```python
from build123d import *

# Parameters (mm, degrees)
F1_DEPTH = 25


with BuildPart() as f1:
    # F0 (on Front) → F1 (new body)
    with BuildSketch(Plane.XZ):
        with BuildLine():
            ThreePointArc((0, 2), (0.5857864376, 0.5857864376), (2, 0))
            Line((2, 0), (14, 0))
            Line((14, 0), (14, 1))
            Line((14, 1), (15, 1))
            Line((15, 1), (15, 6))
            Line((15, 6), (9.95, 6))
            Line((9.95, 6), (9.95, 8.5))
            Line((9.95, 8.5), (13.95, 12.5))
            Line((13.95, 12.5), (19.5, 12.5))
            Line((19.5, 12.5), (20, 13))
            Line((20, 13), (20.5, 12.5))
            Line((20.5, 12.5), (26.05, 12.5))
            Line((26.05, 12.5), (30.05, 8.5))
            Line((30.05, 8.5), (30.05, 6))
            Line((30.05, 6), (25, 6))
            Line((25, 6), (25, 1))
            Line((25, 1), (26, 1))
            Line((26, 1), (26, 0))
            Line((26, 0), (38, 0))
            ThreePointArc((38, 0), (39.4142135624, 0.5857864376), (40, 2))
            Line((40, 2), (40, 14))
            Line((40, 14), (39, 14))
            Line((39, 14), (39, 15))
            Line((39, 15), (34, 15))
            Line((34, 15), (34, 9.95))
            Line((34, 9.95), (31.5, 9.95))
            Line((31.5, 9.95), (27.5, 13.95))
            Line((27.5, 13.95), (27.5, 19.5))
            Line((27.5, 19.5), (27, 20))
            Line((27, 20), (27.5, 20.5))
            Line((27.5, 20.5), (27.5, 26.05))
            Line((27.5, 26.05), (31.5, 30.05))
            Line((31.5, 30.05), (34, 30.05))
            Line((34, 30.05), (34, 25))
            Line((34, 25), (39, 25))
            Line((39, 25), (39, 26))
            Line((39, 26), (40, 26))
            Line((40, 26), (40, 38))
            ThreePointArc((40, 38), (39.4142135624, 39.4142135624), (38, 40))
            Line((38, 40), (26, 40))
            Line((26, 40), (26, 39))
            Line((26, 39), (25, 39))
            Line((25, 39), (25, 34))
            Line((25, 34), (30.05, 34))
            Line((30.05, 34), (30.05, 31.5))
            Line((30.05, 31.5), (26.05, 27.5))
            Line((26.05, 27.5), (20.5, 27.5))
            Line((20.5, 27.5), (20, 27))
            Line((20, 27), (19.5, 27.5))
            Line((19.5, 27.5), (13.95, 27.5))
            Line((13.95, 27.5), (9.95, 31.5))
            Line((9.95, 31.5), (9.95, 34))
            Line((9.95, 34), (15, 34))
            Line((15, 34), (15, 39))
            Line((15, 39), (14, 39))
            Line((14, 39), (14, 40))
            Line((14, 40), (2, 40))
            ThreePointArc((2, 40), (0.5857864376, 39.4142135624), (0, 38))
            Line((0, 38), (0, 26))
            Line((0, 26), (1, 26))
            Line((1, 26), (1, 25))
            Line((1, 25), (6, 25))
            Line((6, 25), (6, 30.05))
            Line((6, 30.05), (8.5, 30.05))
            Line((8.5, 30.05), (12.5, 26.05))
            Line((12.5, 26.05), (12.5, 20.5))
            Line((12.5, 20.5), (13, 20))
            Line((13, 20), (12.5, 19.5))
            Line((12.5, 19.5), (12.5, 13.95))
            Line((12.5, 13.95), (8.5, 9.95))
            Line((8.5, 9.95), (6, 9.95))
            Line((6, 9.95), (6, 15))
            Line((6, 15), (1, 15))
            Line((1, 15), (1, 14))
            Line((1, 14), (0, 14))
            Line((0, 14), (0, 2))
        make_face()
        with BuildLine():
            ThreePointArc((23.8713652105, 23.1642584293), (24.7093962486, 21.6797580105), (25, 20))
            ThreePointArc((25, 20), (24.7093962486, 18.3202419895), (23.8713652105, 16.8357415707))
            ThreePointArc((23.8713652105, 16.8357415707), (23.5355339059, 16.4644660941), (23.1642584293, 16.1286347895))
            ThreePointArc((23.1642584293, 16.1286347895), (20, 15), (16.8357415707, 16.1286347895))
            ThreePointArc((16.8357415707, 16.1286347895), (16.4644660941, 16.4644660941), (16.1286347895, 16.8357415707))
            ThreePointArc((16.1286347895, 16.8357415707), (15, 20), (16.1286347895, 23.1642584293))
            ThreePointArc((16.1286347895, 23.1642584293), (16.4644660941, 23.5355339059), (16.8357415707, 23.8713652105))
            ThreePointArc((16.8357415707, 23.8713652105), (20, 25), (23.1642584293, 23.8713652105))
            ThreePointArc((23.1642584293, 23.8713652105), (23.5355339059, 23.5355339059), (23.8713652105, 23.1642584293))
        make_face(mode=Mode.SUBTRACT)
        with BuildLine():
            Line((17.1969568666, 22.0959363522), (16.1286347895, 23.1642584293))
            ThreePointArc((16.1286347895, 23.1642584293), (15, 20), (16.1286347895, 16.8357415707))
            Line((16.1286347895, 16.8357415707), (17.1969568666, 17.9040636478))
            ThreePointArc((17.1969568666, 17.9040636478), (16.5, 20), (17.1969568666, 22.0959363522))
        make_face()
        with BuildLine():
            ThreePointArc((16.8357415707, 16.1286347895), (20, 15), (23.1642584293, 16.1286347895))
            Line((23.1642584293, 16.1286347895), (22.0959363522, 17.1969568666))
            ThreePointArc((22.0959363522, 17.1969568666), (20, 16.5), (17.9040636478, 17.1969568666))
            Line((17.9040636478, 17.1969568666), (16.8357415707, 16.1286347895))
        make_face()
        with BuildLine():
            ThreePointArc((23.8713652105, 16.8357415707), (24.7093962486, 18.3202419895), (25, 20))
            ThreePointArc((25, 20), (24.7093962486, 21.6797580105), (23.8713652105, 23.1642584293))
            Line((23.8713652105, 23.1642584293), (22.8030431334, 22.0959363522))
            ThreePointArc((22.8030431334, 22.0959363522), (23.3211933824, 21.1043887525), (23.5, 20))
            ThreePointArc((23.5, 20), (23.3211933824, 18.8956112475), (22.8030431334, 17.9040636478))
            Line((22.8030431334, 17.9040636478), (23.8713652105, 16.8357415707))
        make_face()
        with BuildLine():
            Line((22.0959363522, 22.8030431334), (23.1642584293, 23.8713652105))
            ThreePointArc((23.1642584293, 23.8713652105), (20, 25), (16.8357415707, 23.8713652105))
            Line((16.8357415707, 23.8713652105), (17.9040636478, 22.8030431334))
            ThreePointArc((17.9040636478, 22.8030431334), (20, 23.5), (22.0959363522, 22.8030431334))
        make_face()
    extrude(amount=F1_DEPTH)


solid = f1.part
```
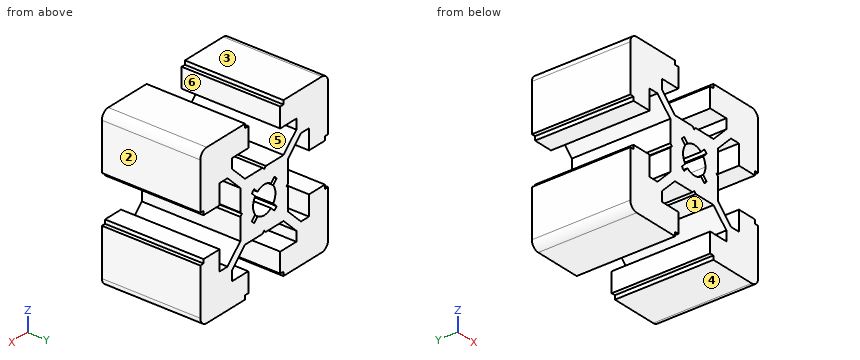
The model under review builds one solid part; all positions refer to its coordinate system, in mm. Face numbers are marked on the shaded views. A direction names the side the tool comes from. Round coordinates to 2 decimals unless told otherwise and drop trailing zeros. Loops run counter-clockwise (first coordinate to the right, second up) from the corner with the lowest first, then second, coordinate; pieces in that order, holes last.
1) Wall thickness on line 1 along X through (y, z) = (-7.5, 14.5); line 2 along X through (y, z) = (-14.75, 7); line 3 along Z through (x, y) = (17, -2.25): over which ranges is each line inside the solid? List them lowest first.
Values follow:
line 1: x = 1 to 6, 12.5 to 27.5, 34 to 39
line 2: x = 0 to 9.95, 30.05 to 40
line 3: z = 12.5 to 16.29, 17.71 to 18.2, 21.8 to 22.29, 23.71 to 27.5
2) The part is to be moulded in two halves that separate along X. For the marked faces 1, 2 and 3, say which applies: pulls with the +X half, pulls with the -X half, needs draft (parallel to the pull), parting line crosses it, or undercut.
Values follow:
face 1: undercut
face 2: pulls with the +X half
face 3: needs draft
3) Consider section A-A on z = 32.5. State the section outline as (x, y) points, then the cut area to 4 significant figures.
Values follow:
outline: (0, -25) - (9.95, -25) - (9.95, 0) - (0, 0) - close; (30.05, -25) - (40, -25) - (40, 0) - (30.05, 0) - close
area: 497.5 mm2
4) Tool access review of the marked faces 4, 5 and 6: name each direction out of +Z, -Z, +X, -X, +Y, -Y from which nothing blocks a thin tool from reaching the whole face with its end or side.
Values follow:
face 4: -Z, +X, -X, +Y, -Y
face 5: +Y, -Y
face 6: +Z, +Y, -Y
5) Clearance check with flat-ended pins moving along their axes: P1, Ø0.5, axis at y = -16.5, z = 0.5, coming from the +X side; P2, Ø0.8, axis at x = 25.5, y = -15.5, coming from the +Z side; P3, Ø2, axis at x = 18.5, y = -5.5, coming from the +Z side; P4, Ø12, axis at x = 20, z = 19, coming from the +Y side. State where each tip first meets the part, or that it passes through.
Values follow:
P1: stops at x = 39.56
P2: stops at z = 39
P3: stops at z = 27.5
P4: stops at y = 0
6) Consider section C-C on z = 11.5. State the section outline as (x, y) points, then the cut area to 3 significant figures.
Values follow:
outline: (0, -25) - (6, -25) - (6, 0) - (0, 0) - close; (10.05, -25) - (12.95, -25) - (12.95, 0) - (10.05, 0) - close; (27.05, -25) - (29.95, -25) - (29.95, 0) - (27.05, 0) - close; (34, -25) - (40, -25) - (40, 0) - (34, 0) - close
area: 445 mm2
7) Consider section D-D on z = 15.5. State the section outline as (x, y) points.
Values follow:
outline: (12.5, -25) - (27.5, -25) - (27.5, 0) - (12.5, 0) - close
8) Consider section B-B on x = 4. State the section outline as (y, z) points.
Values follow:
outline: (-25, 0) - (0, 0) - (0, 15) - (-25, 15) - close; (-25, 25) - (0, 25) - (0, 40) - (-25, 40) - close
